Can you work these out from the drawing? Everything is in mm from the part's minimum corner. Give positions to 0.01 mm unless a question says otherwise; leave off trailing zeros. Order: outer loops, then holes, each group sorted by start corner. A loop starts at its lowest first (then second) coordinate and runs counter-clockwise, first axis right, second up. Notation, with made-up numbers: M -38,28 L 21,28 A26 ccw 21,43 Z; hole C 35,21.25 d11. An arc over 180 degrees is marked long. Answer as a JSON object with one key per item and string values.
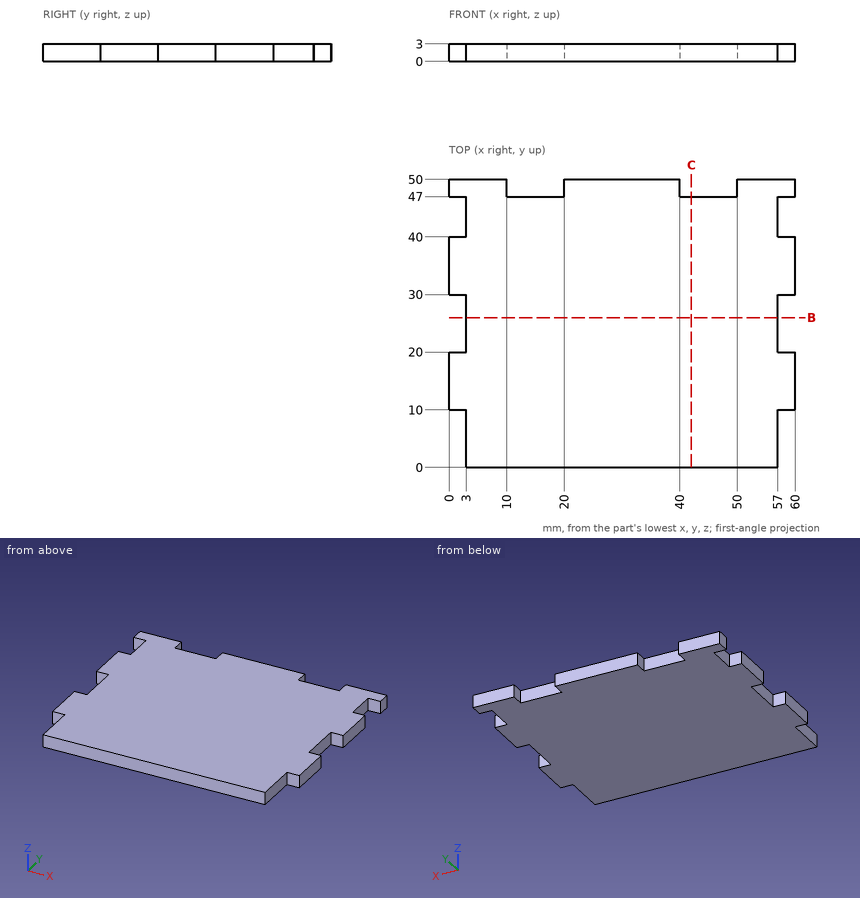
1) I want a section at C-C on x = 42. Write out the boundary of the cut face in (y, z), and give its area (3 significant figures).
Results found:
{"outline": "M 0,0 L 47,0 L 47,3 L 0,3 Z", "area": "141 mm²"}
2) I'm going to push flat-ended pins straight in: pin 1 Ø1.5 at (x, z) = (16.5, 2) entering from +Y; pin 2 Ø1.5 at (x, z) = (1.5, 2) entering from -Y; pin 3 Ø1.5 at (y, z) = (7, 2.5) entering from +X. Where does each tip first touch, or does it pass through?
Results found:
{"pin 1": "stops at y = 47", "pin 2": "stops at y = 10", "pin 3": "stops at x = 57"}
3) I need wall thicknesses on L1, parallel to X at y = 6, z = 2.8; L2, parallel to Y at x = 14, z = 2.05. Which ranges of each line are inside material? Lowest first, please.
Results found:
{"L1": "x = 3 to 57", "L2": "y = 0 to 47"}
4) I want a section at B-B on y = 26. Write out the boundary of the cut face in (x, z).
Results found:
{"outline": "M 3,0 L 57,0 L 57,3 L 3,3 Z"}
